Autodesk Inventor part; units mm, degrees
ref_plane "YZ Plane" through (0, 0, 0) normal (1, 0, 0) x (0, 1, 0)
ref_plane "XZ Plane" through (0, 0, 0) normal (0, 1, 0) x (-1, 0, 0)
ref_plane "XY Plane" through (0, 0, 0) normal (0, 0, 1) x (1, 0, 0)
sketch "Sketch1" plane through (0, 0, 0) normal (0, 0, 1) x (1, 0, 0)
  circle A0 centre (0, 0) radius 1.25
  line L0 (0, 0) -> (8, 0) construction
  circle A1 centre (8, 0) radius 1.25
  arc A2 (1.0526, 2.2676) -> (-1.0526, -2.2676) centre (0, 0) ccw
  arc A3 (9.0526, -2.2676) -> (6.9474, 2.2676) centre (8, 0) ccw
  arc A4 (-1.0526, -2.2676) -> (9.0526, -2.2676) centre (4, 8.6168) ccw
  arc A5 (1.0526, 2.2676) -> (4, 1.6168) centre (4, 8.6168) ccw
  arc A6 (4, 1.6168) -> (6.9474, 2.2676) centre (4, 8.6168) ccw
  dimension "d0" = 2.5
  dimension "d1" = 8
  dimension "d8" = 5
  dimension "d20" = 12
extrude "Extrusion1" add sketch "Sketch1" along normal blind 1.5
properties part number "linkageC_mini"
Part model, mm, in its own coordinate system. A direction names the side the tool comes from. Round coordinates to 2 decimals unless told otherwise and drop trailing zeros. Loops run counter-clockwise (first coordinate to the right, second up) from the corner with the lowest first, then second, coordinate; pieces in that order, holes last. Notation, with made-up numbers: (-8, -14.75) - (39, -14.75) arc R9 ccw to (39, -9.75) - close; hole circle Ø11 at (-14, 33). An arc over 180 degrees is marked (long way). Answer as a JSON object with one key per item and string values.
Item 1: Pull direction Y, two halves, no side cores. Call faces 3 (the face through (10.244, 1.102, 0.74)), 4 (the face through (6.75, -0.05, 0.74)), 5 (the face through (-0.27, 1.22, 0.74)), 6 (the face through (2.512, 1.777, 0.74)): pulls with the +Y half, pulls with the -Y half, needs draft (parallel to the pull), parting line crosses it, or undercut.
Output:
{"face 3": "parting line crosses it", "face 4": "undercut", "face 5": "undercut", "face 6": "pulls with the +Y half"}
Item 2: Band-saw the part on A-A on y = 0.3. List the corners of the cut face in (x, z), plus the area to 3 significant figures.
Output:
{"outline": "(-2.48, 0) - (-1.21, 0) - (-1.21, 1.5) - (-2.48, 1.5) - close; (1.21, 0) - (6.79, 0) - (6.79, 1.5) - (1.21, 1.5) - close; (9.21, 0) - (10.48, 0) - (10.48, 1.5) - (9.21, 1.5) - close", "area": "12.2 mm2"}
Item 3: Band-saw the part on D-D on y = 2. List the corners of the cut face in (x, z).
Output:
{"outline": "(-1.5, 0) - (1.72, 0) - (1.72, 1.5) - (-1.5, 1.5) - close; (6.28, 0) - (9.5, 0) - (9.5, 1.5) - (6.28, 1.5) - close"}
Item 4: Tool access for faces 1 (the face through (4, 0, 1.5)), 2 (the face through (5.53, 1.786, 0.74)): list every direction of +Z, -Z, +X, -X, +Y, -Y with a clear straight run to the whole face (end or side of a thin tool).
Output:
{"face 1": "+Z, +X, -X, +Y, -Y", "face 2": "+Z, -Z, +Y"}
Item 5: Band-saw the part on B-B on x = 0. List the corners of the cut face in (y, z).
Output:
{"outline": "(-2.7, 0) - (-1.25, 0) - (-1.25, 1.5) - (-2.7, 1.5) - close; (1.25, 0) - (2.5, 0) - (2.5, 1.5) - (1.25, 1.5) - close"}
Item 6: Band-saw the part on C-C on z = 0.7. List the corners of the cut face in (x, y).
Output:
{"outline": "(-1.05, -2.27) arc R12 ccw to (9.05, -2.27) arc R2.5 ccw to (6.95, 2.27) arc R7 cw to (4, 1.62) arc R7 cw to (1.05, 2.27) arc R2.5 ccw to start; hole circle Ø2.5 at (0, 0); hole circle Ø2.5 at (8, 0)"}
Item 7: Pin check, flat tip, straight feed: pin 1 (3 mm diameter, centred on x = 8, y = 0, fed in from -Z). Stop position of the tip, or through.
Output:
{"pin 1": "z = 0"}
Item 8: Wall check: L1, parallel to X at y = 0.15, z = 0.2; L2, parallel to X at y = -0.9, z = 0.15; L3, parallel to Y at x = -0.5, z = 0.6. Give the ranges that are in metal, low to high.
Output:
{"L1": "-2.5 to -1.24, 1.24 to 6.76, 9.24 to 10.5", "L2": "-2.33 to -0.87, 0.87 to 7.13, 8.87 to 10.33", "L3": "-2.51 to -1.15, 1.15 to 2.45"}
